from build123d import *

# Parameters (mm, degrees)
SCHIZZO1_W                   = 43
SCHIZZO1_H                   = 39
ESTRUSIONE_ESTRUSIONE1_DEPTH = 3
SCHIZZO2_R                   = 2.5
ESTRUSIONE_ESTRUSIONE2_DEPTH = 3
SCHIZZO3_R                   = 1.25
TAGLIO_ESTRUSIONE1_DEPTH     = 30.639500671
SCHIZZO4_W                   = 30
SCHIZZO4_H                   = 14
TAGLIO_ESTRUSIONE2_DEPTH     = 30.180472923


with BuildPart() as part:
    # Schizzo1 → Estrusione-Estrusione1 (new body)
    with BuildSketch(Plane.XY):
        Rectangle(SCHIZZO1_W, SCHIZZO1_H)
    extrude(amount=ESTRUSIONE_ESTRUSIONE1_DEPTH)

    # Schizzo2 → Estrusione-Estrusione2 (add)
    with BuildSketch(Plane.XY.offset(3)):
        with Locations((19, 17)):
            Circle(SCHIZZO2_R)
        with Locations(Location((-19, 13.25, 0), (0, 0, 180))):
            Circle(SCHIZZO2_R)
        with Locations((19, -17)):
            Circle(SCHIZZO2_R)
        with Locations(Location((-19, -13.25, 0), (0, 0, 180))):
            Circle(SCHIZZO2_R)
    extrude(amount=ESTRUSIONE_ESTRUSIONE2_DEPTH)

    # Schizzo3 → Taglio-Estrusione1 (cut, through all)
    with BuildSketch(Plane.XY.offset(6)):
        with Locations((-19, 13.25)):
            Circle(SCHIZZO3_R)
        with Locations((19, 17)):
            Circle(SCHIZZO3_R)
        with Locations((19, -17)):
            Circle(SCHIZZO3_R)
        with Locations((-19, -13.25)):
            Circle(SCHIZZO3_R)
    extrude(amount=-TAGLIO_ESTRUSIONE1_DEPTH, mode=Mode.SUBTRACT)

    # Schizzo4 → Taglio-Estrusione2 (cut, through all)
    with BuildSketch(Plane.XY.offset(3)):
        with BuildLine():
            Line((-10, 15), (10, 15))
            ThreePointArc((10, 15), (12.5, 12.5), (10, 10))
            Line((10, 10), (-10, 10))
            ThreePointArc((-10, 10), (-12.5, 12.5), (-10, 15))
        make_face()
        with Locations((1.5, 0)):
            Rectangle(SCHIZZO4_W, SCHIZZO4_H)
        with BuildLine():
            Line((-10, -15), (10, -15))
            ThreePointArc((10, -15), (12.5, -12.5), (10, -10))
            Line((10, -10), (-10, -10))
            ThreePointArc((-10, -10), (-12.5, -12.5), (-10, -15))
        make_face()
    extrude(amount=-TAGLIO_ESTRUSIONE2_DEPTH, mode=Mode.SUBTRACT)


solid = part.part
Work out the finished part from the listing and answer in its coordinate system (mm). A direction names the side the tool comes from. Give positions to 0.01 mm unless a question says otherwise; leave off trailing zeros. Loops run counter-clockwise (first coordinate to the right, second up) from the corner with the lowest first, then second, coordinate; pieces in that order, holes last. Notation, with made-up numbers: (4.25, 18.25) - (60.25, 18.25) arc R19 ccw to (60.25, 30.25) - close; hole circle Ø6 at (59.25, 85). An arc over 180 degrees is marked (long way). Answer in a Markdown table with one row per item.
(1) Section D-D (x = 15) is taken. Give the vertices of the cut face in (y, z).
Results list:
| item | result |
|---|---|
| outline | (-19.5, 0) - (-7, 0) - (-7, 3) - (-19.5, 3) - close; (7, 0) - (19.5, 0) - (19.5, 3) - (7, 3) - close |
(2) Section B-B (x = 5) is taken. Give the vertices of the cut face in (y, z).
Results list:
| item | result |
|---|---|
| outline | (-19.5, 0) - (-15, 0) - (-15, 3) - (-19.5, 3) - close; (-10, 0) - (-7, 0) - (-7, 3) - (-10, 3) - close; (7, 0) - (10, 0) - (10, 3) - (7, 3) - close; (15, 0) - (19.5, 0) - (19.5, 3) - (15, 3) - close |
(3) Flat-ended cylindrical pins translate along their axes: pin 1 Ø4 at (x, y) = (-19, -13.25) entering from -Z; pin 2 Ø2 at (x, y) = (-16, -2.5) entering from +Z. Find the tip coordinate at first contact, or state that the pin passes through.
Results list:
| item | result |
|---|---|
| pin 1 | stops at z = 0 |
| pin 2 | stops at z = 3 |
(4) For a pull along X with two mould halves and no side action, classify faces 5 (the face through (-20, -12, 6)), 6 (the face through (16.5, 17.1, 4.5)) as pulls with the +X half, pulls with the -X half, needs draft (parallel to the pull), parting line crosses it, or undercut.
Results list:
| item | result |
|---|---|
| face 5 | needs draft |
| face 6 | undercut |
(5) Section A-A (z = 2) is taken. Give the vertices of the cut face in (x, y), and give its area (3 significant figures).
Results list:
| item | result |
|---|---|
| outline | (-21.5, -19.5) - (21.5, -19.5) - (21.5, 19.5) - (-21.5, 19.5) - close; hole circle Ø2.5 at (-19, -13.25); hole circle Ø2.5 at (-19, 13.25); hole (-13.5, -7) - (16.5, -7) - (16.5, 7) - (-13.5, 7) - close; hole (-10, -15) - (10, -15) arc R2.5 ccw to (10, -10) - (-10, -10) arc R2.5 ccw to start; hole (-10, 10) - (10, 10) arc R2.5 ccw to (10, 15) - (-10, 15) arc R2.5 ccw to start; hole circle Ø2.5 at (19, -17); hole circle Ø2.5 at (19, 17) |
| area | 998 mm² |
(6) A tool of negligible diameter and unlimited length cuts with its end or side. For faces 1 (the face through (21, 19, 3)), 2 (the face through (1, 7, 2)), 3 (the face through (-17.016, 14.771, 4.479)), 4 (the face through (21, -19, 3)), from which of +Z, -Z, +X, -X, +Y, -Y can it reach the whole face along a straight path? Write none if from no direction.
Results list:
| item | result |
|---|---|
| face 1 | +Z, +X, +Y |
| face 2 | +Z, -Z |
| face 3 | +Z |
| face 4 | +Z, +X, -Y |
(7) Section C-C (y = 12.5) is taken. Give the vertices of the cut face in (x, z), and give its area (3 significant figures).
Results list:
| item | result |
|---|---|
| outline | (-21.5, 0) - (-20, 0) - (-20, 6) - (-21.38, 6) - (-21.38, 3) - (-21.5, 3) - close; (-18, 0) - (-12.5, 0) - (-12.5, 3) - (-16.62, 3) - (-16.62, 6) - (-18, 6) - close; (12.5, 0) - (21.5, 0) - (21.5, 3) - (12.5, 3) - close |
| area | 56.3 mm² |
(8) Consider L1, parallel to Y at x = 19, z = 4.5; L2, parallel to Y at x = 18, z = 5.35; L3, parallel to Y at x = -19, z = 2. Determine where each line is inside the solid, lowest interval first. Write a range as [from, to].
Results list:
| item | result |
|---|---|
| L1 | y = [-19.5, -18.25], [-15.75, -14.5], [14.5, 15.75], [18.25, 19.5] |
| L2 | y = [-19.29, -17.75], [-16.25, -14.71], [14.71, 16.25], [17.75, 19.29] |
| L3 | y = [-19.5, -14.5], [-12, 12], [14.5, 19.5] |
